from build123d import *

# Parameters (mm, degrees)
BOSS_EXTRUDE1_DEPTH = 50
FILLET1_R           = 2
FILLET2_R           = 5
FILLET3_R           = 5
FILLET4_R           = 5
FILLET5_R           = 5
FILLET6_R           = 2
CUT_EXTRUDE1_DEPTH  = 50
SKETCH3_R           = 12
CUT_EXTRUDE2_DEPTH  = 50
SKETCH4_R           = 1.5
CUT_EXTRUDE3_DEPTH  = 10


with BuildPart() as part:
    # Sketch1 → Boss-Extrude1 (new body)
    with BuildSketch(Plane.XY):
        Polygon((0, 0), (52, 0), (52, 3), (3, 3), (3, 52), (0, 52), align=None)
    extrude(amount=BOSS_EXTRUDE1_DEPTH)

    # Fillet1
    fillet1_edges = [part.edges().sort_by_distance(p)[0] for p in [
        (0, 0, 25),
    ]]
    fillet(fillet1_edges, radius=FILLET1_R)

    # Fillet2
    fillet2_edges = [part.edges().sort_by_distance(p)[0] for p in [
        (1.5, 52, 50),
    ]]
    fillet(fillet2_edges, radius=FILLET2_R)

    # Fillet3
    fillet3_edges = [part.edges().sort_by_distance(p)[0] for p in [
        (52, 1.5, 50),
    ]]
    fillet(fillet3_edges, radius=FILLET3_R)

    # Fillet4
    fillet4_edges = [part.edges().sort_by_distance(p)[0] for p in [
        (52, 1.5, 0),
    ]]
    fillet(fillet4_edges, radius=FILLET4_R)

    # Fillet5
    fillet5_edges = [part.edges().sort_by_distance(p)[0] for p in [
        (1.5, 52, 0),
    ]]
    fillet(fillet5_edges, radius=FILLET5_R)

    # Fillet6
    fillet6_edges = [part.edges().sort_by_distance(p)[0] for p in [
        (3, 3, 25),
    ]]
    fillet(fillet6_edges, radius=FILLET6_R)

    # Sketch2 → Cut-Extrude1 (cut)
    with BuildSketch(Plane(origin=(0, 3, 0), x_dir=(1, 0, 0), z_dir=(0, 1, 0))):
        with BuildLine():
            Line((39, -43), (13, -43))
            ThreePointArc((13, -43), (10, -40), (13, -37))
            Line((13, -37), (39, -37))
            ThreePointArc((39, -37), (42, -40), (39, -43))
        make_face()
        with BuildLine():
            Line((13, -7), (39, -7))
            ThreePointArc((39, -7), (42, -10), (39, -13))
            Line((39, -13), (13, -13))
            ThreePointArc((13, -13), (10, -10), (13, -7))
        make_face()
    extrude(amount=-CUT_EXTRUDE1_DEPTH, mode=Mode.SUBTRACT)

    # Sketch3 → Cut-Extrude2 (cut)
    with BuildSketch(Plane.ZY):
        with Locations((25, 30)):
            Circle(SKETCH3_R)
    extrude(amount=-CUT_EXTRUDE2_DEPTH, mode=Mode.SUBTRACT)

    # Sketch4 → Cut-Extrude3 (cut)
    with BuildSketch(Plane(origin=(3, 0, 0), x_dir=(0, 0, -1), z_dir=(1, 0, 0))):
        with Locations((-8.85, 46.15)):
            Circle(SKETCH4_R)
        with Locations((-41.15, 46.15)):
            Circle(SKETCH4_R)
        with Locations((-8.85, 13.85)):
            Circle(SKETCH4_R)
        with Locations((-41.15, 13.85)):
            Circle(SKETCH4_R)
    extrude(amount=-CUT_EXTRUDE3_DEPTH, mode=Mode.SUBTRACT)


solid = part.part
Work out the finished part from the listing and answer in its coordinate system (mm). A direction names the side the tool comes from. Round coordinates to 2 decimals unless told otherwise and drop trailing zeros. Loops run counter-clockwise (first coordinate to the right, second up) from the corner with the lowest first, then second, coordinate; pieces in that order, holes last. Notation, with made-up numbers: (41.25, 45) - (84.25, 45) arc R16 cw to (84.25, 59) - close; hole circle Ø1 at (11, 68.5). An arc over 180 degrees is marked (long way). Use one line per item in the form item = value. Start each with the question number.
(1) Find section B-B on z = 25. Determine the outline of the cut face in (x, y).
(2) Find section C-C on y = 46.15. Determine the outline of the cut face in (x, z).
(3) Find section A-A on x = 25.5. Determine the outline of the cut face in (y, z), and give its area (3 significant figures).
(4) Determine the mould class of faces 4 (the face through (1.52, 46.22, 10.35)), 5 (the face through (42, 2, 40)), 6 (the face through (1, 50, 1)) for opening direction Y: +Y half, -Y half, draft (parallel to the pull), parting line (faces both ways), or undercut.
(5) Consider line 1 (Z direction, x = 1, y = 46); line 2 (Y direction, x = 47.5, z = 40); line 3 (Y direction, x = 1.75, z = 25). Determine where each line is inside the solid, lowest interval first.
(6) Which of the six approach directions +Z, -Z, +X, -X, +Y, -Y give full straight-line access (tool end or side, diameter ignored) to faces 1 (the face through (1.52, 14.86, 9.96)), 2 (the face through (42, 2, 10)), 3 (the face through (3, 17.7, 24.6))?
(7) Flat-ended cylindrical pins translate along their axes: P1, Ø5, axis at y = 13.85, z = 41.15, coming from the +X side; P2, Ø1, axis at x = 36, z = 27, coming from the +Y side. Find the tip coordinate at first contact, or state that the pin passes through.
(8) Find section D-D on z = 41. Determine the outline of the cut face in (x, y).
Answer list:
q1.outline = (0, 2) arc R2 ccw to (2, 0) - (52, 0) - (52, 3) - (5, 3) arc R2 cw to (3, 5) - (3, 18) - (0, 18) - close; (0, 42) - (3, 42) - (3, 52) - (0, 52) - close
q2.outline = (0, 0) - (3, 0) - (3, 7.35) - (0, 7.35) - close; (0, 10.35) - (3, 10.35) - (3, 39.65) - (0, 39.65) - close; (0, 42.65) - (3, 42.65) - (3, 50) - (0, 50) - close
q3.outline = (0, 0) - (3, 0) - (3, 7) - (0, 7) - close; (0, 13) - (3, 13) - (3, 37) - (0, 37) - close; (0, 43) - (3, 43) - (3, 50) - (0, 50) - close
q3.area = 114 mm^2
q4.face_4 = undercut
q4.face_5 = draft
q4.face_6 = +Y half
q5.line_1 = 0 to 7.36, 10.34 to 39.66, 42.64 to 50
q5.line_2 = 0 to 3
q5.line_3 = 0.02 to 18, 42 to 52
q6.face_1 = +X, -X
q6.face_2 = +Y, -Y
q6.face_3 = +Z, -Z, +X, +Y
q7.P1 = 3
q7.P2 = 3
q8.outline = (0, 2) arc R2 ccw to (2, 0) - (10.17, 0) - (10.17, 3) - (5, 3) arc R2 cw to (3, 5) - (3, 12.36) - (0, 12.36) - close; (0, 15.34) - (3, 15.34) - (3, 44.66) - (0, 44.66) - close; (0, 47.64) - (3, 47.64) - (3, 52) - (0, 52) - close; (41.83, 0) - (52, 0) - (52, 3) - (41.83, 3) - close
